Design review of the part built by this model. Coordinates are the model's own, in mm. Face numbers are marked on the shaded views. Coordinates: 2 decimals unless noted, no trailing zeros. Write each loop counter-clockwise with the first axis right and the second up, starting at its lowest first coordinate (ties: lowest second). Pieces come first, ordered by that corner, then holes. Notation, with made-up numbers: (-21.75, 29.5) -> (27.25, 29.5) arc R27 ccw to (27.25, 60.5) -> close; hole circle Ø3 at (80.5, 73). An arc over 180 degrees is marked (long way). Return JSON: item names as keys, results as strings. Group by question number.
from build123d import *

# Parameters (mm, degrees)
SKETCH1_R                = 1.5
BOSS_EXTRUDE1_DEPTH      = 1
BOSS_EXTRUDE2_REACH      = 13.64
BOSS_EXTRUDE2_END_RADIUS = 1.5
SKETCH6_R                = 0.375
SKETCH7_R                = 0.375
CUT_EXTRUDE1_DEPTH       = 5


with BuildPart() as part:
    # Sketch1 → Boss-Extrude1 (new, symmetric)
    with BuildSketch(Plane.XY):
        Circle(SKETCH1_R)
    extrude(amount=BOSS_EXTRUDE1_DEPTH, both=True)

    # Boss-Extrude2: up to this cylinder (the profile starts outside it)
    boss_extrude2_end = Plane(origin=(0, 0, 0), z_dir=(0, 0, -1)) * Cylinder(BOSS_EXTRUDE2_END_RADIUS, 31.28, mode=Mode.PRIVATE)
    # Sketch6 → Boss-Extrude2 (add, up to the surface)
    with BuildSketch(Plane(origin=(0, -10, 0), x_dir=(1, 0, 0), z_dir=(0, 1, 0)), mode=Mode.PRIVATE) as boss_extrude2_sk1:
        with Locations(Location((0, 0, 0), (0, 0, 90))):
            Circle(SKETCH6_R)
    boss_extrude2_tool1 = extrude(boss_extrude2_sk1.sketch, amount=BOSS_EXTRUDE2_REACH, mode=Mode.PRIVATE) - boss_extrude2_end
    add(boss_extrude2_tool1.solids().sort_by_distance((0, -10, 0))[0])

    # Sketch7 → Cut-Extrude1 (cut, symmetric)
    with BuildSketch(Plane(origin=(0, 0.78, 1), x_dir=(-1, 0, 0), z_dir=(0, -0.34202014332566943, -0.9396926207859082))):
        with Locations(Location((0, 0, 0), (0, 0, 270))):
            Circle(SKETCH7_R)
    extrude(amount=CUT_EXTRUDE1_DEPTH, both=True, mode=Mode.SUBTRACT)


solid = part.part
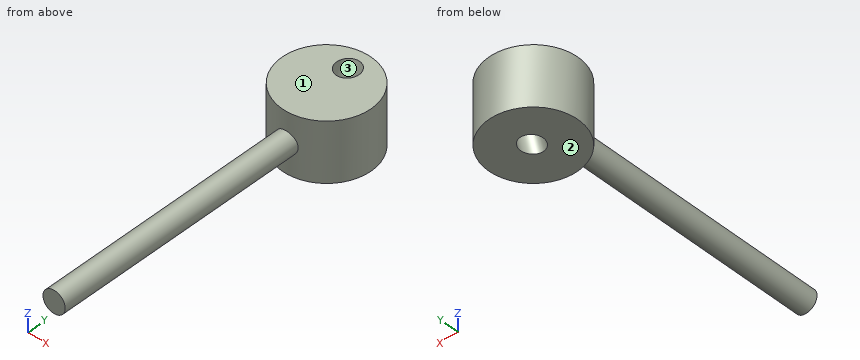
Q1. We need section A-A on x = 0. Write out the cut boundary in (y, z) (3 decimals).
Q2. We need section D-D on x = -0.5. Write out the cut boundary in (y, z), plus the area to 3 significant figures.
Q3. Wall thickness on L1, parallel to X at y = -3, z = 0.05; L2, parallel to Y at x = 0.25, z = 0.1; L3, parallel to X at y = 1, z = 0.7: over which ranges is each line inside the solid? List them lowest first.
Q4. We need section C-C on x = 0.6. Write out the cut boundary in (y, z).
Q5. For P1, Ø1, axis at x = 0.5, y = -5, coming from the +Z side (3 decimals), flat-tipped, find the tip position at first contact; note if it passes through.
Q6. The part is to be moulded in two halves that separate along Z. For the marked faces 1, 2 and 3, say which applies: +Z half, -Z half, draft (parallel to the pull), parting line (faces both ways), or undercut.
Q7. We need section B-B on y = -3.75. Write out the cut boundary in (x, z) (3 decimals), plus the area to 3 significant figures.
Findings below:
{
 "1": {"outline": "(-10, -0.375) -> (-1.5, -0.375) -> (-1.5, -1) -> (-0.347, -1) -> (0.381, 1) -> (-1.5, 1) -> (-1.5, 0.375) -> (-10, 0.375) -> close; (0.451, -1) -> (1.5, -1) -> (1.5, 1) -> (1.179, 1) -> close"},
 "2": {"outline": "(-1.41, -1) -> (1.41, -1) -> (1.41, 1) -> (-1.41, 1) -> close", "area": "5.66 mm^2"},
 "3": {"L1": "x = -0.37 to 0.37", "L2": "y = -10 to 0.15, 0.75 to 1.48", "L3": "x = -1.12 to -0.21, 0.21 to 1.12"},
 "4": {"outline": "(-1.37, -1) -> (1.37, -1) -> (1.37, 1) -> (-1.37, 1) -> close"},
 "5": {"P1": "stops at z = 0.375"},
 "6": {"face 1": "+Z half", "face 2": "-Z half", "face 3": "undercut"},
 "7": {"outline": "circle Ø0.75 at (0, 0)", "area": "0.442 mm^2"}
}
